Input: part model. Units: mm. Frame: model coordinates. Face numbers are marked on the shaded views. A direction names the side the tool comes from. Give positions to 0.01 mm unless a question says otherwise; leave off trailing zeros. Loops run counter-clockwise (first coordinate to the right, second up) from the corner with the lowest first, then second, coordinate; pieces in that order, holes last. Notation, with made-up numbers: (-33.5, 0) -> (-29.5, 0) arc R29 cw to (-29.5, 33) -> close; hole circle Ø6 at (85, -29.5). An arc over 180 degrees is marked (long way). Use CSV: the item, a comma, the result in double quotes.
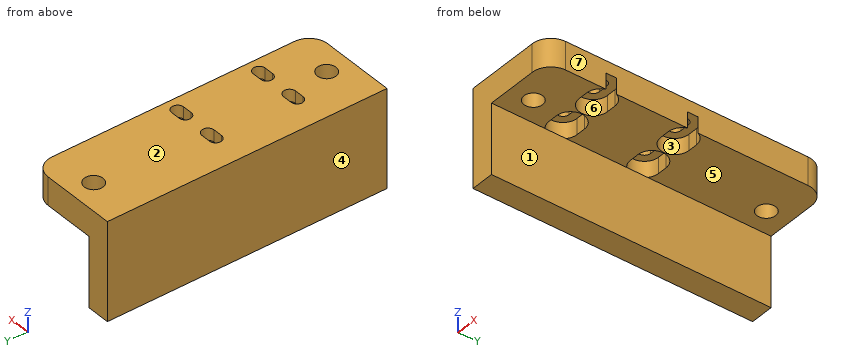
```python
from build123d import *

# Parameters (mm, degrees)
SKETCH1_W                                     = 25.4
SKETCH1_H                                     = 76.2
BOSS_EXTRUDE1_DEPTH                           = 7.62
F_10_CLEARANCE_HOLE1_D                        = 5.1054
F_10_CLEARANCE_HOLE1_DEPTH                    = 25.4
F_10_CLEARANCE_HOLE1_TIP                      = 1.533816902
CBORE_SLOT_FOR_4_SOCKET_HEAD_CAP_SCREW1_DEPTH = 4.318
CBORE_START                                   = 4.318
CBORE_SLOT_FOR_4_SOCKET_HEAD_CAP_SC_3_DEPTH   = 3.302
FILLET1_R                                     = 5.08
SKETCH8_W                                     = 6.35
SKETCH8_H                                     = 76.2
BOSS_EXTRUDE2_DEPTH                           = 19.05


# Read off the part's stored shape, not the designer's step: CBORE SLOT for #4 Socket Head Cap Screw1
with BuildPart() as part:
    # Sketch1 → Boss-Extrude1 (new body)
    with BuildSketch(Plane.XY):
        Rectangle(SKETCH1_W, SKETCH1_H)
    extrude(amount=BOSS_EXTRUDE1_DEPTH)

    # #10 Clearance Hole1
    with Locations(Plane.XY.offset(7.62)):
        with Locations((0, 31.75), (0, -31.75)):
            Hole(F_10_CLEARANCE_HOLE1_D / 2, depth=F_10_CLEARANCE_HOLE1_DEPTH)
            with Locations((0, 0, -(F_10_CLEARANCE_HOLE1_DEPTH + F_10_CLEARANCE_HOLE1_TIP / 2))):  # 118° drill point
                Cone(0, F_10_CLEARANCE_HOLE1_D / 2, F_10_CLEARANCE_HOLE1_TIP, mode=Mode.SUBTRACT)

    # CBORE SLOT for _4 Socket Head Cap Sc 2 → CBORE SLOT for #4 Socket Head Cap Screw1 (cut)
    with BuildSketch(Plane.XY):
        with BuildLine():
            Line((12.7, -22.053863194), (12.7, -19.221136806))
            ThreePointArc((12.7, -19.221136806), (11.298437111, -17.48215186), (9.16305, -16.8275))
            Line((9.16305, -16.8275), (6.58495, -16.8275))
            ThreePointArc((6.58495, -16.8275), (2.77495, -20.6375), (6.58495, -24.4475))
            Line((6.58495, -24.4475), (9.16305, -24.4475))
            ThreePointArc((9.16305, -24.4475), (11.298437111, -23.79284814), (12.7, -22.053863194))
        make_face()
        with BuildLine():
            ThreePointArc((12.7, 3.003863194), (11.298437111, 4.74284814), (9.16305, 5.3975))
            Line((9.16305, 5.3975), (6.58495, 5.3975))
            ThreePointArc((6.58495, 5.3975), (2.77495, 1.5875), (6.58495, -2.2225))
            Line((6.58495, -2.2225), (9.16305, -2.2225))
            ThreePointArc((9.16305, -2.2225), (11.298437111, -1.56784814), (12.7, 0.171136806))
            Line((12.7, 0.171136806), (12.7, 3.003863194))
        make_face()
        with BuildLine():
            ThreePointArc((-3.82905, 5.3975), (-7.63905, 1.5875), (-3.82905, -2.2225))
            Line((-3.82905, -2.2225), (-1.25095, -2.2225))
            ThreePointArc((-1.25095, -2.2225), (2.55905, 1.5875), (-1.25095, 5.3975))
            Line((-1.25095, 5.3975), (-3.82905, 5.3975))
        make_face()
        with BuildLine():
            ThreePointArc((-3.82905, -16.8275), (-7.63905, -20.6375), (-3.82905, -24.4475))
            Line((-3.82905, -24.4475), (-1.25095, -24.4475))
            ThreePointArc((-1.25095, -24.4475), (2.55905, -20.6375), (-1.25095, -16.8275))
            Line((-1.25095, -16.8275), (-3.82905, -16.8275))
        make_face()
    extrude(amount=CBORE_SLOT_FOR_4_SOCKET_HEAD_CAP_SCREW1_DEPTH, mode=Mode.SUBTRACT)

    # CBORE SLOT for _4 Socket Head Cap Sc 3 o → CBORE SLOT for _4 Socket Head Cap Sc 3 (cut)
    with BuildSketch(Plane.XY.offset(CBORE_START)):
        with BuildLine():
            ThreePointArc((9.16305, -0.04445), (10.795, 1.5875), (9.16305, 3.21945))
            Line((9.16305, 3.21945), (6.58495, 3.21945))
            ThreePointArc((6.58495, 3.21945), (4.953, 1.5875), (6.58495, -0.04445))
            Line((6.58495, -0.04445), (9.16305, -0.04445))
        make_face()
        with BuildLine():
            ThreePointArc((-3.82905, 3.21945), (-5.461, 1.5875), (-3.82905, -0.04445))
            Line((-3.82905, -0.04445), (-1.25095, -0.04445))
            ThreePointArc((-1.25095, -0.04445), (0.381, 1.5875), (-1.25095, 3.21945))
            Line((-1.25095, 3.21945), (-3.82905, 3.21945))
        make_face()
        with BuildLine():
            ThreePointArc((9.16305, -22.26945), (10.795, -20.6375), (9.16305, -19.00555))
            Line((9.16305, -19.00555), (6.58495, -19.00555))
            ThreePointArc((6.58495, -19.00555), (4.953, -20.6375), (6.58495, -22.26945))
            Line((6.58495, -22.26945), (9.16305, -22.26945))
        make_face()
        with BuildLine():
            ThreePointArc((-3.82905, -19.00555), (-5.461, -20.6375), (-3.82905, -22.26945))
            Line((-3.82905, -22.26945), (-1.25095, -22.26945))
            ThreePointArc((-1.25095, -22.26945), (0.381, -20.6375), (-1.25095, -19.00555))
            Line((-1.25095, -19.00555), (-3.82905, -19.00555))
        make_face()
    extrude(amount=CBORE_SLOT_FOR_4_SOCKET_HEAD_CAP_SC_3_DEPTH, mode=Mode.SUBTRACT)

    # Fillet1
    fillet1_edges = [part.edges().sort_by_distance(p)[0] for p in [
        (12.7, 38.1, 3.81),
        (12.7, -38.1, 3.81),
    ]]
    fillet(fillet1_edges, radius=FILLET1_R)

    # Sketch8 → Boss-Extrude2 (add)
    with BuildSketch(Plane(origin=(0, 0, 0), x_dir=(-1, 0, 0), z_dir=(0, 0, -1))):
        with Locations((9.525, 0)):
            Rectangle(SKETCH8_W, SKETCH8_H)
    extrude(amount=BOSS_EXTRUDE2_DEPTH)


solid = part.part
```
1) Section query C-C (z = -14.75). Return loops of the section in (x, y), then the cut area to 3 significant figures.
From the geometry:
outline,"(-12.7, -38.1) -> (-6.35, -38.1) -> (-6.35, 38.1) -> (-12.7, 38.1) -> close"
area,"484 mm^2"
2) Contact query for flat-ended pins moving along their axis: pin 1 (6 mm diameter, centred on x = -5, y = -21.5, fed in from -Z); pin 2 (0.8 mm diameter, centred on x = 8.5, z = 5.5, fed in from +Y); pin 3 (8.5 mm diameter, centred on x = 9.5, y = -22.5, fed in from -Z); pin 4 (3 mm diameter, centred on y = 18.5, z = -12.5, fed in from +X). Output: stop coordinate, or through.
From the geometry:
pin 1,"stops at z = -19.05"
pin 2,"stops at y = 38.08"
pin 3,"stops at z = 0"
pin 4,"stops at x = -6.35"
3) Mould query, pull axis X, two halves, no side actions, for the marked faces 4, 5, 6 and 7. Classes: pulls with the +X half, pulls with the -X half, needs draft (parallel to the pull), parting line crosses it, or undercut.
From the geometry:
face 4,"pulls with the -X half"
face 5,"needs draft"
face 6,"undercut"
face 7,"pulls with the +X half"
4) Ray query, line 1 (Y direction, x = -2.75, z = 6); line 2 (Y direction, x = -3.5, z = 4.25); line 3 (Y direction, x = 0, z = 4). Return the intervals inside material, ascending.
From the geometry:
line 1,"y = -38.1 to -22.27, -19.01 to -0.04, 3.22 to 38.1"
line 2,"y = -38.1 to -24.45, -16.83 to -2.22, 5.4 to 38.1"
line 3,"y = -38.1 to -34.3, -29.2 to -24.24, -17.04 to -2.01, 5.19 to 29.2, 34.3 to 38.1"
5) Reachability of the marked faces 1, 2 and 3 from +Z, -Z, +X, -X, +Y, -Y: full face, straight path, thin tool, end or side. Return the list, or none.
From the geometry:
face 1,"-Z, +X, +Y, -Y"
face 2,"+Z, +X, -X, +Y, -Y"
face 3,"-Z"
6) Section query A-A (y = -31.75). Return loops of the section in (x, z).
From the geometry:
outline,"(-12.7, -19.05) -> (-6.35, -19.05) -> (-6.35, 0) -> (-2.55, 0) -> (-2.55, 7.62) -> (-12.7, 7.62) -> close; (2.55, 0) -> (12.7, 0) -> (12.7, 7.62) -> (2.55, 7.62) -> close"
7) Section query B-B (y = -5.5). Return loops of the section in (x, z), then the cut area to 3 significant figures.
From the geometry:
outline,"(-12.7, -19.05) -> (-6.35, -19.05) -> (-6.35, 0) -> (12.7, 0) -> (12.7, 7.62) -> (-12.7, 7.62) -> close"
area,"315 mm^2"
